The drawing under review shows one solid part. Ordinate dimensions are in mm from its lowest x, y, z. Give positions to 0.01 mm unless a question says otherwise; leave off trailing zeros. Order: outer loops, then holes, each group sorted by start corner. A loop starts at its lowest first (then second) coordinate and runs counter-clockwise, first axis right, second up. Notation, with made-up numbers: (0, 26.25) - (43, 26.25) arc R7 cw to (43, 33.25) - close; hole circle Ø8 at (56, 66). An arc over 180 degrees is marked (long way). Use CSV: the item, a comma, the result in double quotes. Start each with the question number.
1. For pin 1 (1.6 mm diameter, centred on x = 19.05, y = 3.175, fed in from +Z), flat-tipped, find the tip position at first contact; note if it passes through.
2. Take a section at B-B, the plane x = 19.05. State the section outline as (y, z) points, then the cut area to 3 significant figures.
3. Take a section at C-C, the plane y = 0.75. State the section outline as (x, z) points.
4. To check wall thickness, follow line 1 (Y direction, x = 19.05, z = 6); line 2 (X direction, y = 2.5, z = 3.75); line 3 (X direction, y = 3.5, z = 3). State the ranges of each line that lie inside material, in increasing order. Write a range as [from, to].
5. Draft analysis for pull direction X (two halves, no side actions). For the marked faces 1, 2 and 3, state which applies: released by +X, released by -X, zero draft, split by the parting line, or undercut.
6. Take a section at A-A, the plane z = 5.5. Count the separate pieces of the cut face and the enclosed holes in it, then the cut area to 3 significant figures.
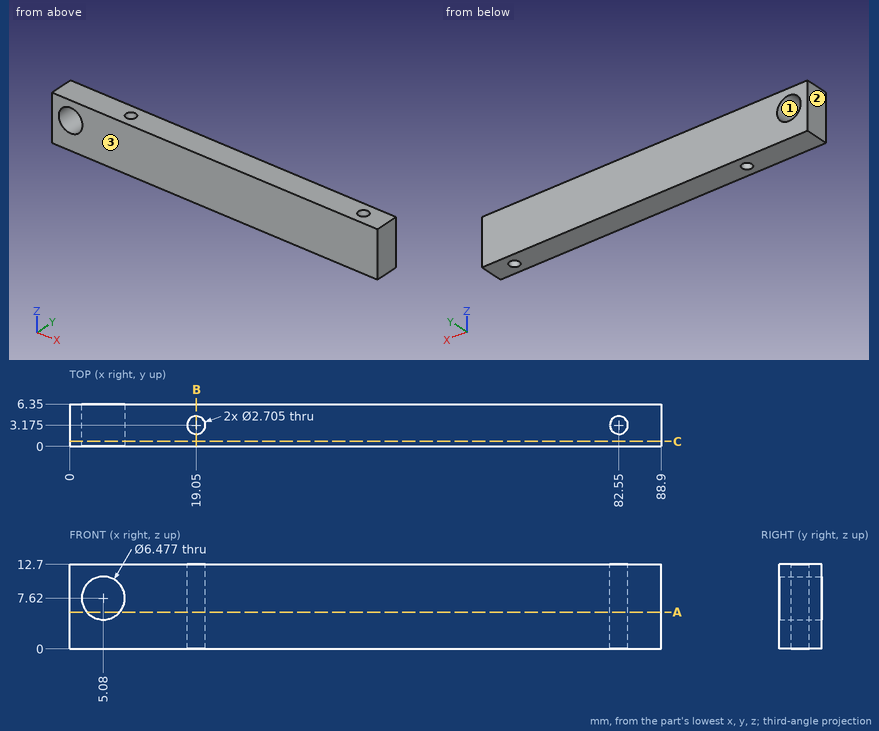
Determined:
1,pin 1,"passes through"
2,outline,"(0, 0) - (1.82, 0) - (1.82, 12.7) - (0, 12.7) - close; (4.53, 0) - (6.35, 0) - (6.35, 12.7) - (4.53, 12.7) - close"
2,area,"46.3 mm²"
3,outline,"(0, 0) - (88.9, 0) - (88.9, 12.7) - (0, 12.7) - close; hole circle Ø6.48 at (5.08, 7.62)"
4,line 1,"y = [0, 1.82], [4.53, 6.35]"
4,line 2,"x = [0, 17.88], [20.22, 81.38], [83.72, 88.9]"
4,line 3,"x = [0, 17.74], [20.36, 81.24], [83.86, 88.9]"
5,face 1,"undercut"
5,face 2,"released by -X"
5,face 3,"zero draft"
6,separate pieces,"2"
6,enclosed holes,"2"
6,area,"522 mm²"
